Verification items for this drawing (mm, ordinates from the low corner). Round coordinates to 2 decimals unless told otherwise and drop trailing zeros. Order: outer loops, then holes, each group sorted by start corner. A loop starts at its lowest first (then second) coordinate and runs counter-clockwise, first axis right, second up. Notation, with made-up numbers: (49.25, -35) - (90.25, -35) arc R24 ccw to (90.25, 3) - close; hole circle Ø2 at (6, 55). An arc over 180 degrees is marked (long way). One line per question, with ' | ' between items. Start each with the question number.
Q1. Sectioned sample at C-C, the plane x = 6. Enter the section's corners in (y, z), then the cut area to 3 significant figures.
Q2. Sectioned sample at D-D, the plane y = 29.5. Enter the section's corners in (x, z).
Q3. Gauge pin test, flat ends, axial feed: P1, Ø3, axis at x = 6.17, y = 10.75, coming from the -Z side; P2, Ø1.5, axis at y = 22.5, z = 4.5, coming from the +X side; P3, Ø2, axis at y = 21, z = 4.5, coming from the -X side; P4, Ø3, axis at x = 13, z = 1.5, coming from the -Y side (1 decimal). Record the tip position at first contact, or that the pin passes through.
Q4. Sectioned sample at A-A, the plane y = 10.75. Enter the section's corners in (x, z) (1 decimal).
Q5. Mould release check, pull along Y, two halves, no side actions. Record for the marked faces 1, 2 and 3: +Y half, -Y half, draft (parallel to the pull), parting line (faces both ways), or undercut.
Q6. Sectioned sample at B-B, the plane z = 3.75. Give the number of separate pieces and of enclosed holes in the cut face, then the cut area to 3 significant figures.
Q7. Material ranges on line 1 along Y through (x, z) = (17, 3.5); line 2 along X through (y, z) = (29, 4.5) (1 decimal); line 3 along Y through (x, z) = (18.5, 2.5), recorded low to high.
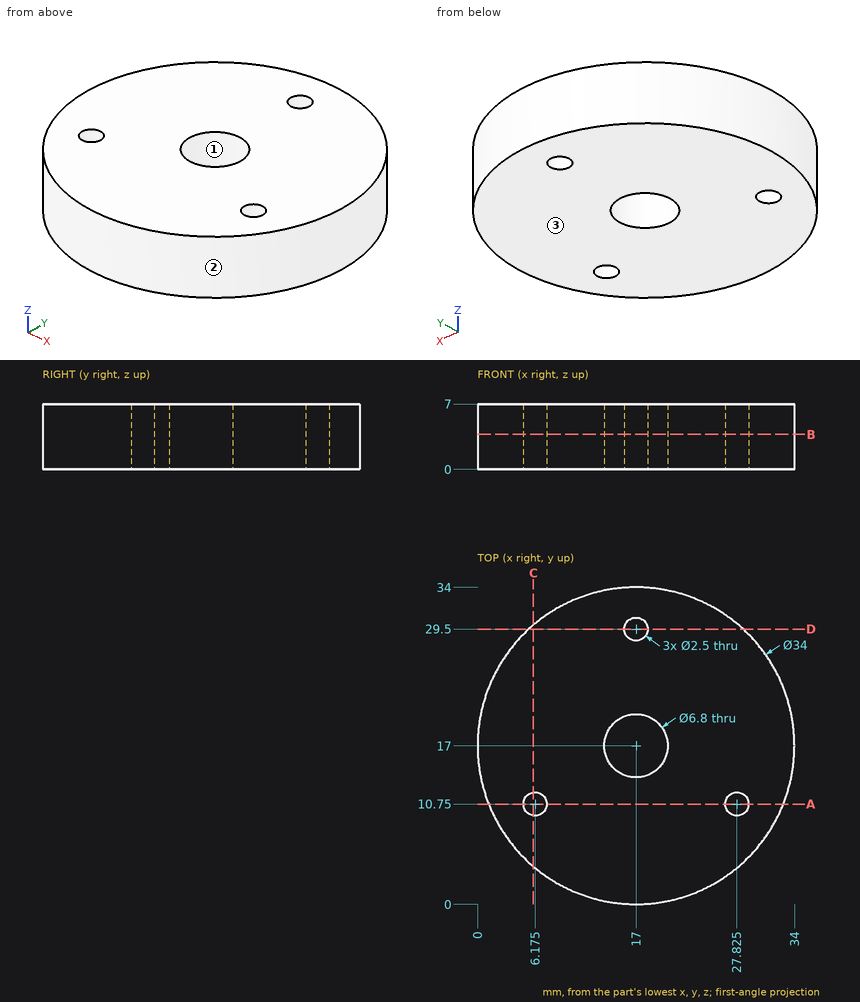
Determined:
1) outline: (4.04, 0) - (9.51, 0) - (9.51, 7) - (4.04, 7) - close; (11.99, 0) - (29.96, 0) - (29.96, 7) - (11.99, 7) - close | area: 164 mm2
2) outline: (5.48, 0) - (15.75, 0) - (15.75, 7) - (5.48, 7) - close; (18.25, 0) - (28.52, 0) - (28.52, 7) - (18.25, 7) - close
3) P1: stops at z = 0 | P2: stops at x = 33.32 | P3: stops at x = 0.27 | P4: stops at y = 0.2
4) outline: (1.2, 0) - (4.9, 0) - (4.9, 7) - (1.2, 7) - close; (7.4, 0) - (26.6, 0) - (26.6, 7) - (7.4, 7) - close; (29.1, 0) - (32.8, 0) - (32.8, 7) - (29.1, 7) - close
5) face 1: undercut | face 2: parting line | face 3: draft
6) separate pieces: 1 | enclosed holes: 4 | area: 857 mm2
7) line 1: y = 0 to 13.6, 20.4 to 28.25, 30.75 to 34 | line 2: x = 5 to 15.9, 18.1 to 29 | line 3: y = 0.07 to 13.95, 20.05 to 33.93
